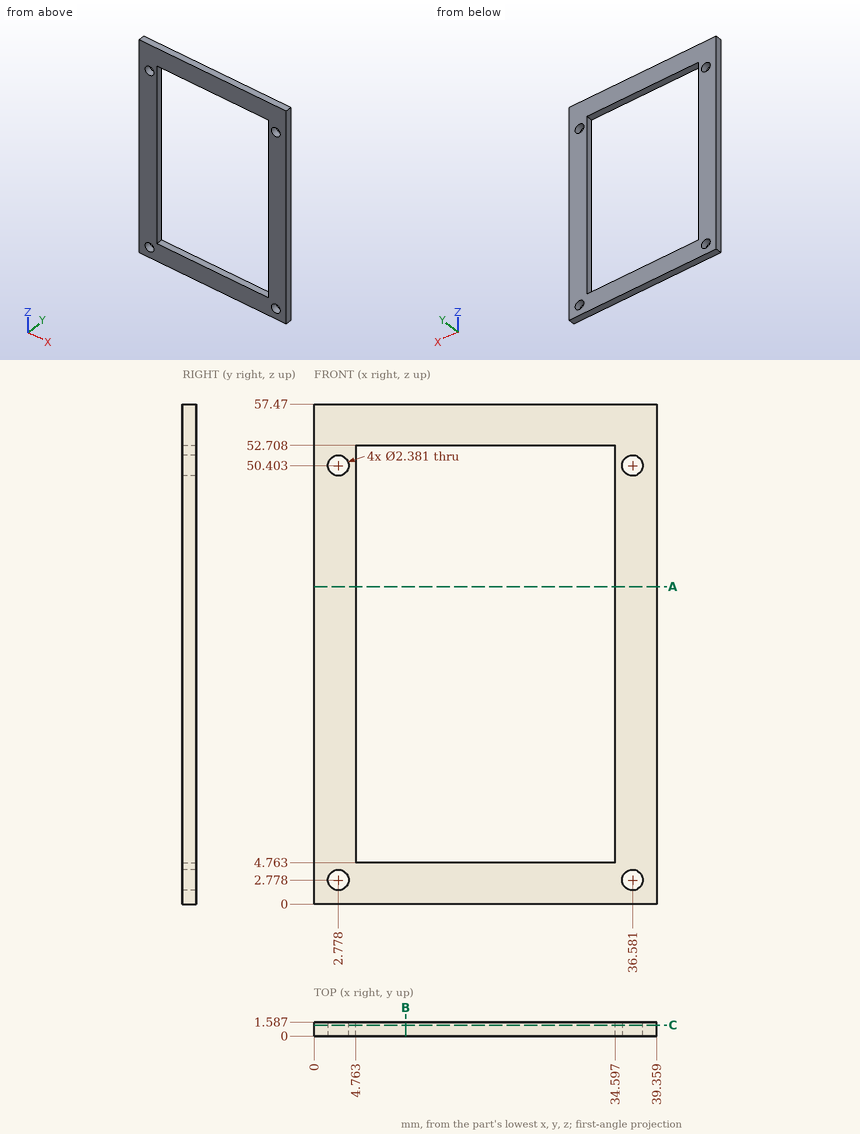
Print and shaded views of the part. All mm, measured from the part's lowest x, y and z. Round coordinates to 2 decimals unless told otherwise and drop trailing zeros. Write each loop counter-clockwise with the first axis right and the second up, starting at its lowest first coordinate (ties: lowest second). Pieces come first, ordered by that corner, then holes. Notation, with made-up numbers: (-7, 62.5) -> (20, 62.5) arc R27 cw to (20, 80.5) -> close; hole circle Ø5 at (2.25, 54.25). An arc over 180 degrees is marked (long way). Answer in a Markdown table with one row per item. Add a question column.
Item 1: Drop a flat-ended pin along its axis: pin 1 Ø1.4 at (x, z) = (36.58, 2.78) entering from +Y. Give the stop position or say it passes through.
Item 2: Saw through at A-A, the plane z = 36.5. Write the cut outline in (x, y), then the cut area to 3 significant figures.
Item 3: Drill centre lines: line 1 (X direction, y = 0.35, z = 19.5); line 2 (Z direction, x = 32, y = 1.35). Where is each one in solid material? Low to high. Write a range as from..to.
Item 4: Saw through at C-C, the plane y = 1.25. Write the cut outline in (x, z).
Item 5: Saw through at B-B, the plane x = 10.5. Write the cut outline in (y, z), then the cut area to 3 significant figures.
Findings below:
| question | item | result |
|---|---|---|
| 1 | pin 1 | passes through |
| 2 | outline | (0, 0) -> (4.76, 0) -> (4.76, 1.59) -> (0, 1.59) -> close; (34.6, 0) -> (39.36, 0) -> (39.36, 1.59) -> (34.6, 1.59) -> close |
| 2 | area | 15.1 mm^2 |
| 3 | line 1 | x = 0..4.76, 34.6..39.36 |
| 3 | line 2 | z = 0..4.76, 52.71..57.47 |
| 4 | outline | (0, 0) -> (39.36, 0) -> (39.36, 57.47) -> (0, 57.47) -> close; hole circle Ø2.38 at (2.78, 2.78); hole circle Ø2.38 at (2.78, 50.4); hole (4.76, 4.76) -> (34.6, 4.76) -> (34.6, 52.71) -> (4.76, 52.71) -> close; hole circle Ø2.38 at (36.58, 2.78); hole circle Ø2.38 at (36.58, 50.4) |
| 5 | outline | (0, 0) -> (1.59, 0) -> (1.59, 4.76) -> (0, 4.76) -> close; (0, 52.71) -> (1.59, 52.71) -> (1.59, 57.47) -> (0, 57.47) -> close |
| 5 | area | 15.1 mm^2 |
